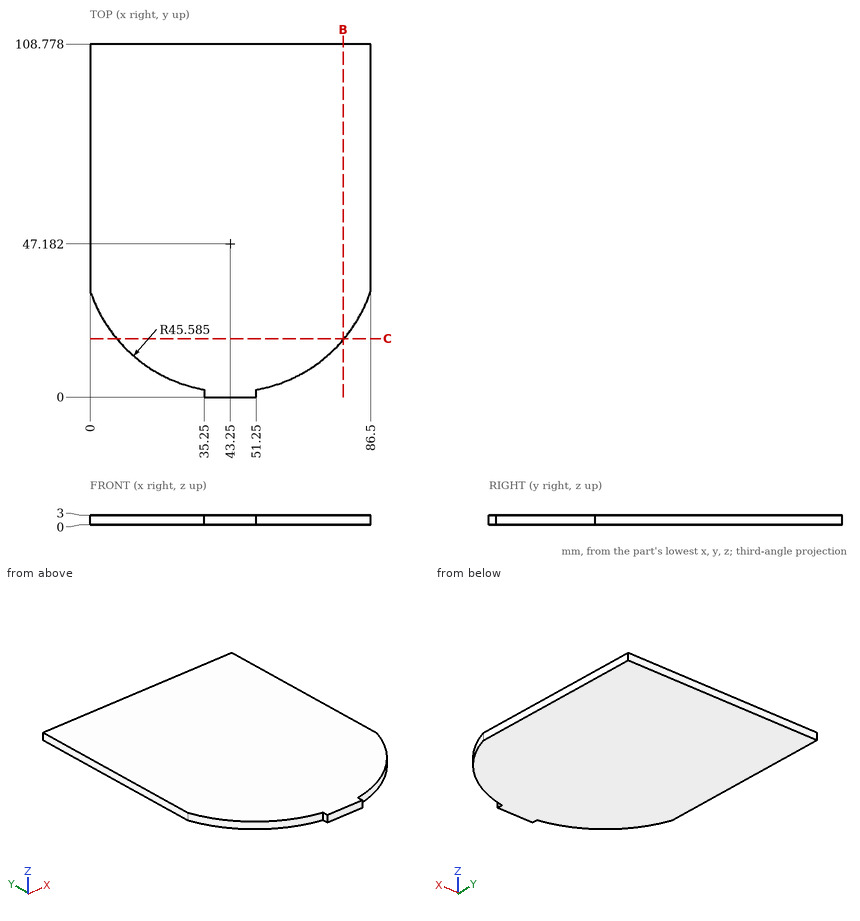
Input: dimensioned drawing with shaded views. Units: mm. Origin: part minimum x, y, z. Coordinates: 2 decimals unless noted, no trailing zeros. Loops run counter-clockwise (first coordinate to the right, second up) from the corner with the lowest first, then second, coordinate; pieces in that order, holes last.
Q1. Line query: line 1 along X through (y, z) = (16, 1.85); line 2 along X through (y, z) = (8.5, 0.5); line 3 along Y through (x, z) = (77.5, 1.1). Output: solid intervals per line, ascending.
Results are:
line 1: x = 10 to 76.5
line 2: x = 19.13 to 67.37
line 3: y = 17.1 to 108.78
Q2. Section C-C, the plane y = 18. Return the cut outline in (x, z).
Results are:
outline: (8.23, 0) - (78.27, 0) - (78.27, 3) - (8.23, 3) - close
Q3. Contact query for a flat-ended pin moving along its axis: pin 1 (1.2 mm diameter, centred on y = 1, z = 2, fed in from -X). Output: stop coordinate, or through.
Results are:
pin 1: stops at x = 35.25
Q4. Section B-B, the plane x = 78. Return the cut outline in (y, z).
Results are:
outline: (17.68, 0) - (108.78, 0) - (108.78, 3) - (17.68, 3) - close
